```python
from build123d import *

# Parameters (mm, degrees)
F0_W      = 3.81
F0_H      = 6.35
F0_W_2    = 91.186
F0_H_2    = 125.476
F0_H_3    = 35.306
F0_W_3    = 52.324
F0_W_4    = 82.042
F0_W_5    = 85.852
F0_H_4    = 42.418
F0_H_5    = 143.002
F0_H_6    = 3.81
F1_DEPTH  = 114.3
F2_SIZE2  = 40.64
F2_SIZE   = 50.8
F4_DEPTH  = 101.6
F6_DEPTH  = 245.872
F8_DEPTH  = 133.35
F9_W      = 38.1
F9_H      = 43.866105608
F10_DEPTH = 88.9
F11_W     = 6.35
F11_H     = 6.35
F12_DEPTH = 88.9
F13_W     = 42.164
F13_H     = 38.1
F14_DEPTH = 4.318
F15_SIZE2 = 3.81
F15_SIZE  = 15.24
F16_SIZE2 = 13.97
F16_SIZE  = 3.81
F17_DEPTH = 5.08
F18_W     = 42.164
F18_H     = 38.1
F19_DEPTH = 4.318
F20_SIZE2 = 13.97
F20_SIZE  = 3.81
F21_SIZE2 = 13.97
F21_SIZE  = 3.81
F18_W_2   = 50.8
F22_DEPTH = 5.08
F18_W_3   = 30.48
F23_DEPTH = 5.08
F24_W     = 31.75
F24_H     = 38.1
F25_DEPTH = 5.08


with BuildPart() as f1:
    # F0 (on Top) → F1 (new body)
    with BuildSketch(Plane.XY):
        Polygon((150.876, 63.754), (245.872, 63.754), (245.872, 243.586), (0, 243.586), (0, 0), (150.876, 0), align=None)
        Polygon((6.35, 201.93), (6.35, 237.236), (88.392, 237.236), (92.202, 237.236), (144.526, 237.236), (148.336, 237.236), (239.522, 237.236), (239.522, 201.93), (239.522, 195.58), (239.522, 70.104), (148.336, 70.104), (144.526, 70.104), (144.526, 6.35), (96.012, 6.35), (92.202, 6.35), (6.35, 6.35), (6.35, 149.352), (6.35, 153.162), (6.35, 195.58), align=None, mode=Mode.SUBTRACT)
        with Locations((146.431, 198.755)):
            Rectangle(F0_W, F0_H)
        with Locations((193.929, 132.842)):
            Rectangle(F0_W_2, F0_H_2)
        with Locations((193.929, 219.583)):
            Rectangle(F0_W_2, F0_H_3)
        with Locations((118.364, 219.583)):
            Rectangle(F0_W_3, F0_H_3)
        with Locations((47.371, 219.583)):
            Rectangle(F0_W_4, F0_H_3)
        with Locations((49.276, 174.371)):
            Rectangle(F0_W_5, F0_H_4)
        Polygon((144.526, 195.58), (96.012, 195.58), (96.012, 6.35), (144.526, 6.35), (144.526, 70.104), align=None)
        with Locations((146.431, 132.842)):
            Rectangle(F0_W, F0_H_2)
        with Locations((49.276, 77.851)):
            Rectangle(F0_W_5, F0_H_5)
        Polygon((96.012, 195.58), (92.202, 195.58), (92.202, 153.162), (92.202, 149.352), (92.202, 6.35), (96.012, 6.35), align=None)
        with Locations((49.276, 151.257)):
            Rectangle(F0_W_5, F0_H_6)
        with Locations((193.929, 198.755)):
            Rectangle(F0_W_2, F0_H)
        Polygon((88.392, 201.93), (6.35, 201.93), (6.35, 195.58), (92.202, 195.58), (96.012, 195.58), (144.526, 195.58), (144.526, 201.93), (92.202, 201.93), align=None)
        with Locations((146.431, 219.583)):
            Rectangle(F0_W, F0_H_3)
        with Locations((90.297, 219.583)):
            Rectangle(F0_W, F0_H_3)
    extrude(amount=F1_DEPTH)

    # F2
    f2_edges = [f1.edges().sort_by_distance(p)[0] for p in [
        (122.936, 243.586, 114.3),
    ]]
    f2_side = f1.faces().sort_by_distance((122.936, 243.586, 57.15))[0]
    chamfer(f2_edges, length=F2_SIZE, length2=F2_SIZE2, reference=f2_side)

    # F3 (on face) → F4 (join)
    with BuildSketch(Plane.XY.offset(114.3)):
        Polygon((5.8203e-06, 0), (150.876, 0), (150.876, 63.754), (245.872, 63.754), (245.872, 202.946), (5.8203e-06, 202.946), align=None)
    extrude(amount=F4_DEPTH)

    # F5 (on face) → F6 (join, through all)
    with BuildSketch(Plane.YZ.offset(245.872)):
        Polygon((133.35, 292.1), (63.754, 215.9), (202.946, 215.9), align=None)
    extrude(amount=-F6_DEPTH)

    # F7 (on face) → F8 (join, through all)
    with BuildSketch(Plane.XZ):
        Polygon((75.438, 279.4), (0, 215.9), (150.876, 215.9), align=None)
    extrude(amount=-F8_DEPTH)

    # F9 (on face) → F10 (cut)
    with BuildSketch(Plane(origin=(0, 0, 0), x_dir=(1, 0, 0), z_dir=(0, 0, -1))):
        with Locations((131.826, -21.933052804)):
            Rectangle(F9_W, F9_H)
    extrude(amount=-F10_DEPTH, mode=Mode.SUBTRACT)

    # F11 (on face) → F12 (join, through all)
    with BuildSketch(Plane(origin=(0, 0, 88.9), x_dir=(1, 0, 0), z_dir=(0, 0, -1))):
        with Locations((147.701, -3.175)):
            Rectangle(F11_W, F11_H)
    extrude(amount=F12_DEPTH)

    # F13 (on face) → F14 (join)
    with BuildSketch(Plane.XZ.offset(-63.754)):
        with Locations((194.564, 44.45)):
            Rectangle(F13_W, F13_H)
    extrude(amount=F14_DEPTH)

    # F15
    f15_edges = [f1.edges().sort_by_distance(p)[0] for p in [
        (215.646, 59.436, 44.45),
    ]]
    f15_side = f1.faces().sort_by_distance((194.564, 59.436, 44.45))[0]
    chamfer(f15_edges, length=F15_SIZE, length2=F15_SIZE2, reference=f15_side)

    # F16
    f16_edges = [f1.edges().sort_by_distance(p)[0] for p in [
        (173.482, 59.436, 44.45),
    ]]
    f16_side = f1.faces().sort_by_distance((173.482, 61.595, 44.45))[0]
    chamfer(f16_edges, length=F16_SIZE, length2=F16_SIZE2, reference=f16_side)

    # F13 (on face) → F17 (cut)
    with BuildSketch(Plane.XZ.offset(-63.754)):
        with Locations((195.58, 146.05)):
            Rectangle(F13_W, F13_H)
    extrude(amount=-F17_DEPTH, mode=Mode.SUBTRACT)

    # F18 (on face) → F19 (join)
    with BuildSketch(Plane.XZ):
        with Locations((51.562, 44.45)):
            Rectangle(F18_W, F18_H)
    extrude(amount=F19_DEPTH)

    # F20
    f20_edges = [f1.edges().sort_by_distance(p)[0] for p in [
        (72.644, -4.318, 44.45),
    ]]
    f20_side = f1.faces().sort_by_distance((72.644, -2.159, 44.45))[0]
    chamfer(f20_edges, length=F20_SIZE, length2=F20_SIZE2, reference=f20_side)

    # F21
    f21_edges = [f1.edges().sort_by_distance(p)[0] for p in [
        (30.48, -4.318, 44.45),
    ]]
    f21_side = f1.faces().sort_by_distance((30.48, -2.159, 44.45))[0]
    chamfer(f21_edges, length=F21_SIZE, length2=F21_SIZE2, reference=f21_side)

    # F18 (on face) → F22 (cut)
    with BuildSketch(Plane.XZ):
        with Locations((40.64, 146.05)):
            Rectangle(F18_W_2, F18_H)
    extrude(amount=-F22_DEPTH, mode=Mode.SUBTRACT)

    # F18 (on face) → F23 (cut)
    with BuildSketch(Plane.XZ):
        with Locations((109.22, 146.05)):
            Rectangle(F18_W_3, F18_H)
    extrude(amount=-F23_DEPTH, mode=Mode.SUBTRACT)

    # F24 (on face) → F25 (cut)
    with BuildSketch(Plane.YZ.offset(150.876)):
        with Locations((26.289, 145.9290999826)):
            Rectangle(F24_W, F24_H)
    extrude(amount=-F25_DEPTH, mode=Mode.SUBTRACT)


solid = f1.part
```
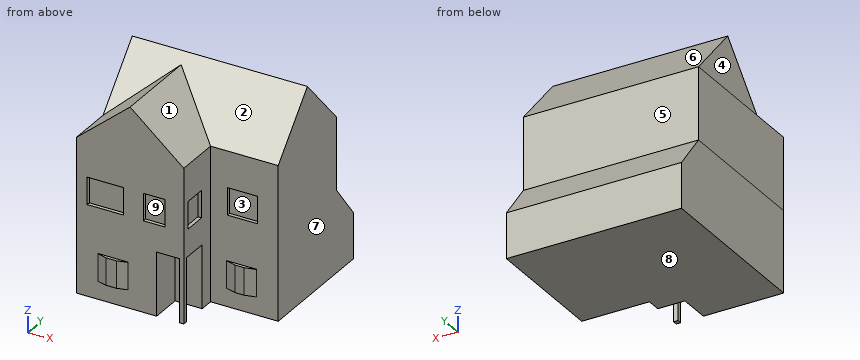
Input: part model. Units: mm. Frame: model coordinates. Face numbers are marked on the shaded views. A direction names the side the tool comes from. Round coordinates to 2 decimals unless told otherwise and drop trailing zeros. Write each loop counter-clockwise with the first axis right and the second up, starting at its lowest first coordinate (ties: lowest second). Pieces come first, ordered by that corner, then holes. Notation, with made-up numbers: M 74,-40 L 127,-40 A24 cw 127,-14 Z; hole C 71,18.5 d11. An arc over 180 degrees is marked long. Write each question's results on one line, items separated by ' | '.
Q1. Line query: line 1 along Y through (x, z) = (121.5, 191.5); line 2 along Y through (x, z) = (228, 31); line 3 along Z through (x, y) = (80, 66.5). Output: solid intervals per line, ascending.
Results:
line 1: y = 0 to 202.95 | line 2: y = 63.75 to 243.59 | line 3: z = 0 to 275.56
Q2. Draft query along Z for the marked faces 6, 7, 8 and 9. Return one class per face: released by +Z, released by -Z, zero draft, split by the parting line, or undercut.
Results:
face 6: released by +Z | face 7: zero draft | face 8: released by -Z | face 9: undercut
Q3. Section query D-D (x = 230.5). Return loops of the section in (y, z), and give its area (3 significant figures).
Results:
outline: M 63.75,0 L 243.59,0 L 243.59,63.5 L 202.95,114.3 L 202.95,215.9 L 133.35,292.1 L 63.75,215.9 Z | area: 39,000 mm^2
Q4. Section query B-B (z = 134). Return loops of the section in (x, y), and give its area (3 significant figures).
Results:
outline: M 0,0 L 15.24,0 L 15.24,5.08 L 66.04,5.08 L 66.04,0 L 93.98,0 L 93.98,5.08 L 124.46,5.08 L 124.46,0 L 150.88,0 L 150.88,10.41 L 145.8,10.41 L 145.8,42.16 L 150.88,42.16 L 150.88,63.75 L 174.5,63.75 L 174.5,68.83 L 216.66,68.83 L 216.66,63.75 L 245.87,63.75 L 245.87,202.95 L 0,202.95 Z | area: 43,100 mm^2
Q5. Section query A-A (z = 34.5). Return loops of the section in (x, y).
Results:
outline: M 0,0 L 30.48,0 L 30.48,-0.51 L 44.45,-4.32 L 58.67,-4.32 L 72.64,-0.51 L 72.64,0 L 112.78,0 L 112.78,43.87 L 150.88,43.87 L 150.88,63.75 L 173.48,63.75 L 173.48,63.25 L 187.45,59.44 L 200.41,59.44 L 215.65,63.25 L 215.65,63.75 L 245.87,63.75 L 245.87,243.59 L 0,243.59 Z; M 144.53,0 L 150.88,0 L 150.88,6.35 L 144.53,6.35 Z
Q6. Access query for the marked faces 1, 2, 3, 4 and 5. Directions: +Z, -Z, +X, -X, +Y, -Y. A direction counts if a zero-diameter tool reaches every point of the face in a straight line with its end or side. Return the directions, or none.
Results:
face 1: +Z, +X, -Y | face 2: +Z, -Y | face 3: -Y | face 4: +Z, -Z, -X, +Y, -Y | face 5: +Z, +X, -X, +Y
Q7. Pin query (flat end, axial travel): P1, Ø1.5, axis at x = 91.5, z = 163.5, coming from the -Y side; P2, Ø4, axis at x = 196, z = 42.5, coming from the -Y side; P3, Ø3, axis at x = 196.5, z = 110, coming from the +Y side. Return the tip coordinate at first contact, or that it passes through.
Results:
P1: stops at y = 0 | P2: stops at y = 59.44 | P3: stops at y = 207.59
